from build123d import *

# Parameters (mm, degrees)
F0_W     = 15
F0_H     = 20
F1_DEPTH = 15
F2_W     = 220
F2_H     = 125
F2_W_2   = 15
F2_H_2   = 55
F3_DEPTH = 5
F4_W     = 180
F4_H     = 10
F5_DEPTH = 10


with BuildPart() as f1:
    # F0 (on Front) → F1 (new body)
    with BuildSketch(Plane.XZ):
        with Locations((12.5, 17.5)):
            Rectangle(F0_W, F0_H)
        with Locations((12.5, -17.5)):
            Rectangle(F0_W, F0_H)
        Polygon((5, 7.5), (-20, 7.5), (-20, -7.5), (5, -7.5), (20, -7.5), (20, 7.5), align=None)
    extrude(amount=F1_DEPTH)

    # F2 (on face) → F3 (join)
    with BuildSketch(Plane.YZ.offset(20)):
        with Locations((-7.5, 0)):
            Rectangle(F2_W, F2_H)
        with Locations((-7.5, 0)):
            Rectangle(F2_W_2, F2_H_2, mode=Mode.SUBTRACT)
        with Locations((-7.5, 0)):
            Rectangle(F2_W_2, F2_H_2)
    extrude(amount=F3_DEPTH)

    # F4 (on face) → F5 (join)
    with BuildSketch(Plane.YZ.offset(25)):
        with Locations((-7.5, -57.5)):
            Rectangle(F4_W, F4_H)
    extrude(amount=F5_DEPTH)


solid = f1.part
Check sheet for the modelled part. Datum: model origin and axes. Units: mm. A direction names the side the tool comes from. Round coordinates to 2 decimals unless told otherwise and drop trailing zeros. Loops run counter-clockwise (first coordinate to the right, second up) from the corner with the lowest first, then second, coordinate; pieces in that order, holes last. Notation, with made-up numbers: (45, 31.25) -> (68, 31.25) arc R13 cw to (68, 48.25) -> close; hole circle Ø6 at (89, 36.25). An arc over 180 degrees is marked (long way). Put each result on its own line as item: value. Start each with the question number.
1. Gauge pin test, flat ends, axial feed: pin 1 (1 mm diameter, centred on y = -56.5, z = 2, fed in from +X); pin 2 (16.5 mm diameter, centred on x = -7, y = -8.5, fed in from -Z); pin 3 (4.5 mm diameter, centred on x = -11.5, y = -5, fed in from +Z). Record the tip position at first contact, or that the pin passes through.
2. Access from +Z, -Z, +X, -X, +Y, -Y to the whole of each face (thin tool, end or side, straight path). Record for faces 1 (the face through (30, -9, -52.5)), 2 (the face through (12, -7, 27.5)), 3 (the face through (12, -7, -27.5)), 4 (the face through (4, -15, 0)).
3. Section check C-C (x = 11.5). Enter the section's corners in (y, z).
4. Section check B-B (y = 13). Enter the section's corners in (x, z).
5. Section check D-D (z = 17). Enter the section's corners in (x, y).
6. Scan lines: probe 1 along X at (y, z) = (53, -57); probe 2 along X at (y, z) = (87.5, 31); probe 3 along Y at (x, z) = (19, 16). Record each from-to range of solid material in increasing order.
7. Section check A-A (z = 3). Enter the section's corners in (x, y).
Findings:
1. pin 1: stops at x = 25
1. pin 2: stops at z = -7.5
1. pin 3: stops at z = 7.5
2. face 1: +Z, +X, +Y, -Y
2. face 2: +Z, -X, +Y, -Y
2. face 3: -Z, -X, +Y, -Y
2. face 4: +Z, -Z, -X, -Y
3. outline: (-15, -27.5) -> (0, -27.5) -> (0, 27.5) -> (-15, 27.5) -> close
4. outline: (20, -62.5) -> (35, -62.5) -> (35, -52.5) -> (25, -52.5) -> (25, 62.5) -> (20, 62.5) -> close
5. outline: (5, -15) -> (20, -15) -> (20, -117.5) -> (25, -117.5) -> (25, 102.5) -> (20, 102.5) -> (20, 0) -> (5, 0) -> close
6. probe 1: x = 20 to 35
6. probe 2: x = 20 to 25
6. probe 3: y = -15 to 0
7. outline: (-20, -15) -> (20, -15) -> (20, -117.5) -> (25, -117.5) -> (25, 102.5) -> (20, 102.5) -> (20, 0) -> (-20, 0) -> close
